```python
from build123d import *

# Parameters (mm, degrees)
SKETCH1_R                      = 22.5
BOSS_EXTRUDE1_DEPTH            = 2.5
M3_CLEARANCE_HOLE1_D           = 3.4
M3_CLEARANCE_HOLE1_CSINK_D     = 3.45
M3_CLEARANCE_HOLE1_CSINK_ANGLE = 90
SKETCH6_R                      = 10
BOSS_EXTRUDE2_DEPTH            = 6
HOLE2_D                        = 4.5
HOLE2_CBORE_D                  = 5.2
HOLE2_CBORE_DEPTH              = 1.5


with BuildPart() as part:
    # Sketch1 → Boss-Extrude1 (new body)
    with BuildSketch(Plane.XY):
        Circle(SKETCH1_R)
    extrude(amount=BOSS_EXTRUDE1_DEPTH)

    # M3 Clearance Hole1 (through all)
    with Locations(Plane.XY.offset(2.5)):
        with Locations((-14.289419162, 8.25), (14.289419162, 8.25), (0, -16.5)):
            CounterSinkHole(M3_CLEARANCE_HOLE1_D / 2, M3_CLEARANCE_HOLE1_CSINK_D / 2, counter_sink_angle=M3_CLEARANCE_HOLE1_CSINK_ANGLE)

    # Sketch6 → Boss-Extrude2 (add)
    with BuildSketch(Plane.XY.offset(2.5)):
        Circle(SKETCH6_R)
    extrude(amount=BOSS_EXTRUDE2_DEPTH)

    # Hole2 (through all)
    with Locations(Plane.XY.offset(8.5)):
        with Locations((0, 5), (0, -5)):
            CounterBoreHole(HOLE2_D / 2, HOLE2_CBORE_D / 2, HOLE2_CBORE_DEPTH)


solid = part.part
```
Here's how the part is built. I have some questions about the finished solid (model axes, mm). A direction names the side the tool comes from. Give positions to 0.01 mm unless a question says otherwise; leave off trailing zeros. Write each loop counter-clockwise with the first axis right and the second up, starting at its lowest first coordinate (ties: lowest second). Pieces come first, ordered by that corner, then holes. Notation, with made-up numbers: (65.5, 34.25) -> (80.5, 34.25) arc R32 ccw to (80.5, 70.25) -> close; hole circle Ø11 at (-35.75, -40). An arc over 180 degrees is marked (long way). Write each question's results on one line, items separated by ' | '.
Item 1: Suppose I cut it at A-A on x = 0. Give the number of separate pieces and of enclosed holes in the cut face, plus the area to 3 significant figures.
Output:
separate pieces: 4 | enclosed holes: 0 | area: 145 mm^2
Item 2: For pin 1 Ø1 at (x, y) = (11.5, -2) entering from +Z; pin 2 Ø2.5 at (x, y) = (0, 5) entering from +Z; pin 3 Ø2.5 at (x, y) = (-1, 4.5) entering from +Z; pin 4 Ø2 at (y, z) = (-1.5, 4.5) entering from -X, each with a flat end and sliding along its axis, tell me the tip position at first contact or that it passes through.
Output:
pin 1: stops at z = 2.5 | pin 2: passes through | pin 3: stops at z = 7 | pin 4: stops at x = -9.99
Item 3: We'd pull the mould along X, two halves only. Please class faces 3 (the face through (0, 0, 0)), 4 (the face through (1.2, -7.307, 7.76)), 5 (the face through (-2.17, -9.76, 5.46)): pulls with the +X half, pulls with the -X half, needs draft (parallel to the pull), parting line crosses it, or undercut.
Output:
face 3: needs draft | face 4: undercut | face 5: parting line crosses it
Item 4: Suppose I cut it at B-B on y = -16.5. Write out the boundary of the cut face in (x, z) (3 decimals).
Output:
outline: (-15.297, 0) -> (-1.7, 0) -> (-1.7, 2.475) -> (-1.725, 2.5) -> (-15.297, 2.5) -> close; (1.7, 0) -> (15.297, 0) -> (15.297, 2.5) -> (1.725, 2.5) -> (1.7, 2.475) -> close
Item 5: Suppose I cut it at C-C on y = 8.25. Write out the boundary of the cut face in (x, z) (3 decimals).
Output:
outline: (-20.933, 0) -> (-15.989, 0) -> (-15.989, 2.475) -> (-16.014, 2.5) -> (-20.933, 2.5) -> close; (-12.589, 0) -> (12.589, 0) -> (12.589, 2.475) -> (12.564, 2.5) -> (5.651, 2.5) -> (5.651, 8.5) -> (-5.651, 8.5) -> (-5.651, 2.5) -> (-12.564, 2.5) -> (-12.589, 2.475) -> close; (15.989, 0) -> (20.933, 0) -> (20.933, 2.5) -> (16.014, 2.5) -> (15.989, 2.475) -> close
Item 6: On a 3-axis mill with a long thin cutter (end or side, diameter ignored), from which of +Z, -Z, +X, -X, +Y, -Y can I reach the whole of each face in a straight line? I mean faces 1 (the face through (5, -10, 2.5)), 2 (the face through (0, 0, 8.5)). Say none if no direction works.
Output:
face 1: +Z | face 2: +Z, +X, -X, +Y, -Y
Item 7: Suppose I cut it at D-D on y = 0. Write out the boundary of the cut face in (x, z).
Output:
outline: (-22.5, 0) -> (22.5, 0) -> (22.5, 2.5) -> (10, 2.5) -> (10, 8.5) -> (-10, 8.5) -> (-10, 2.5) -> (-22.5, 2.5) -> close
Item 8: If I drill on L1, parallel to Y at x = 0, z = 5; L2, parallel to Y at x = 0, z = 1.55; L3, parallel to Y at x = 0, z = 7.6, over which ranges is the centre line in solid material (lowest first)?
Output:
L1: y = -10 to -7.25, -2.75 to 2.75, 7.25 to 10 | L2: y = -22.5 to -18.2, -14.8 to -7.25, -2.75 to 2.75, 7.25 to 22.5 | L3: y = -10 to -7.6, -2.4 to 2.4, 7.6 to 10
